Autodesk Inventor part; units mm, degrees
ref_plane "YZ Plane" through (0, 0, 0) normal (1, 0, 0) x (0, 1, 0)
ref_plane "XZ Plane" through (0, 0, 0) normal (0, 1, 0) x (-1, 0, 0)
ref_plane "XY Plane" through (0, 0, 0) normal (0, 0, 1) x (1, 0, 0)
sketch "Sketch1" plane through (0, 0, 0) normal (0, 1, 0) x (-1, 0, 0)
  line L0 (13.5, 14) -> (13.5, 15)
  line L1 (13.5, 15) -> (17.5, 15)
  line L2 (17.5, 15) -> (17.5, 20)
  line L3 (17.5, 20) -> (0, 20)
  line L4 (0, 20) -> (0, 0)
  line L5 (13.5, 14) -> (12.5, 14)
  line L6 (12.5, 14) -> (12.5, 0)
  line L7 (12.5, 0) -> (0, 0)
  dimension "d1" = 27
  dimension "d2" = 35
  dimension "d3" = 1
  dimension "d4" = 5
  dimension "d28" = 25
  dimension "d29" = 14
revolve "Revolution1" add sketch "Sketch1" angle 360 about axis through (0, 0, 20) along (0, 0, -1)
sketch "Sketch2" plane through (0, 0, 20) normal (0, 0, 1) x (1, 0, 0)
  point P0 (0, 0)
  point P1 (0, 9.5)
  dimension "d6" = 9.5
hole "Hole1" at (0, 9.5, 20) direction (0, 0, -1) diameter 3.4 end through all counterbore diameter 6.5 counterbore depth 4
pattern_circular "Circular Pattern1" count 6 over 360 about axis through (0, 0, -10) along (0, 0, -1) of "Hole1"
sketch "Sketch3" plane through (0, 0, 20) normal (0, 0, 1) x (1, 0, 0)
  point P0 (0, 0)
  point P1 (14, 0)
  dimension "d17" = 14
hole "Hole2" at (14, 0, 20) direction (0, 0, -1) diameter 2.459 end through all
pattern_circular "Circular Pattern2" count 6 over 360 about axis through (0, 0, -10) along (0, 0, 1) of "Hole2"
equation "\"d28\" = bearing_61705_inner"
equation "\"bearing_61807_inner\" = 35"
equation "\"bearing_61807_outer\" = 47.1"
equation "\"bearing_61814_outer\" = 90.1"
equation "\"bearing_61705_outer\" = 32.1"
equation "\"bearing_61705_inner\" = 25"
equation "\"M3_adjustable\" = 3.2"
equation "\"bearing_606_outer\" = 17.1"
equation "\"gearbox_35_outer\" = 32.3"
properties part number "405-output disk"
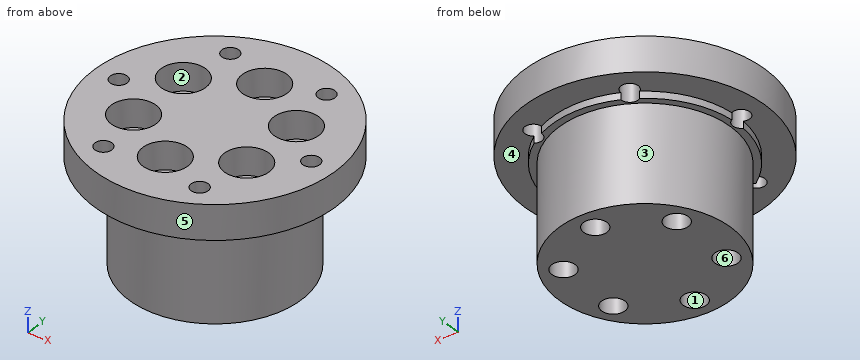
CAD build for the part. Positions are in the model's coordinates, mm. Face numbers are marked on the shaded views. A direction names the side the tool comes from. Give positions to 0.01 mm unless a question says otherwise; leave off trailing zeros. Loops run counter-clockwise (first coordinate to the right, second up) from the corner with the lowest first, then second, coordinate; pieces in that order, holes last. Notation, with made-up numbers: M -15.5,-38.75 L 20.5,-38.75 A18 ccw 20.5,-14.75 Z; hole C 56,11.5 d4. An arc over 180 degrees is marked long. Use one line per item in the form item = value.
Item 1: Flat gauge pins, fed straight in: pin 1 (2 mm diameter, centred on x = 7, y = -12.12, fed in from -Z); pin 2 (2 mm diameter, centred on y = 10, z = 14.5, fed in from -X); pin 3 (2 mm diameter, centred on x = -9.5, y = -5.5, fed in from +Z); pin 4 (3 mm diameter, centred on x = -1, z = 9.5, fed in from -Y). Where does each tip first touch, or does it go through?
Determined:
pin_1 = through
pin_2 = -14.93
pin_3 = 16
pin_4 = -12.5
Item 2: Slice it at A-A (x = 0). List the corners of the cut face in (y, z).
Determined:
outline = M -17.5,15 L -13.5,15 L -13.5,14 L -12.5,14 L -12.5,0 L -11.2,0 L -11.2,16 L -12.75,16 L -12.75,20 L -17.5,20 Z; M -7.8,0 L 7.8,0 L 7.8,16 L 6.25,16 L 6.25,20 L -6.25,20 L -6.25,16 L -7.8,16 Z; M 11.2,0 L 12.5,0 L 12.5,14 L 13.5,14 L 13.5,15 L 17.5,15 L 17.5,20 L 12.75,20 L 12.75,16 L 11.2,16 Z
Item 3: Two-plate mould, pull along X, no slides. Class the marked faces 4, 5 and 6: pulls with the +X half, pulls with the -X half, needs draft (parallel to the pull), parting line crosses it, or undercut.
Determined:
face_4 = needs draft
face_5 = parting line crosses it
face_6 = undercut
Item 4: Slice it at C-C (x = 14). List the corners of the cut face in (y, z), plus the area to 3 significant figures.
Determined:
outline = M -10.5,15 L -1.23,15 L -1.23,20 L -10.5,20 Z; M 1.23,15 L 10.5,15 L 10.5,20 L 1.23,20 Z
area = 92.7 mm2
Item 5: Which spindle directions (+Z, -Z, +X, -X, +Y, -Y) get a long thin tool onto all of the face, cutting with end or side? Do the marked faces 1, 2 and 3. Say none if no direction does.
Determined:
face_1 = +Z, -Z
face_2 = +Z
face_3 = -Z
Item 6: Slice it at B-B (y = 0). List the corners of the cut face in (x, z).
Determined:
outline = M -17.5,15 L -15.23,15 L -15.23,20 L -17.5,20 Z; M -12.77,14 L -12.5,14 L -12.5,0 L 12.5,0 L 12.5,14 L 12.77,14 L 12.77,20 L -12.77,20 Z; M 15.23,15 L 17.5,15 L 17.5,20 L 15.23,20 Z
Item 7: Slice it at D-D (z = 10.5). List the corners of the cut face in (x, y) (3 decimals), plus the area to 3 significant figures.
Determined:
outline = C 0,0 d25; hole C -8.227,-4.75 d3.4; hole C -8.227,4.75 d3.4; hole C 0,-9.5 d3.4; hole C 0,9.5 d3.4; hole C 8.227,-4.75 d3.4; hole C 8.227,4.75 d3.4
area = 436 mm2
Item 8: Drill centre lines: probe 1 along Y at (x, z) = (-7, 13.75); probe 2 along X at (y, z) = (4.75, 10.25); probe 3 along Y at (x, z) = (9, 10). Where is each one in solid material? Low to high. Write a range as from..to.
Determined:
probe_1 = -10.36..-5.93, -3.57..3.57, 5.93..10.36
probe_2 = -11.56..-9.93, -6.53..6.53, 9.93..11.56
probe_3 = -8.67..-6.26, -3.24..3.24, 6.26..8.67
